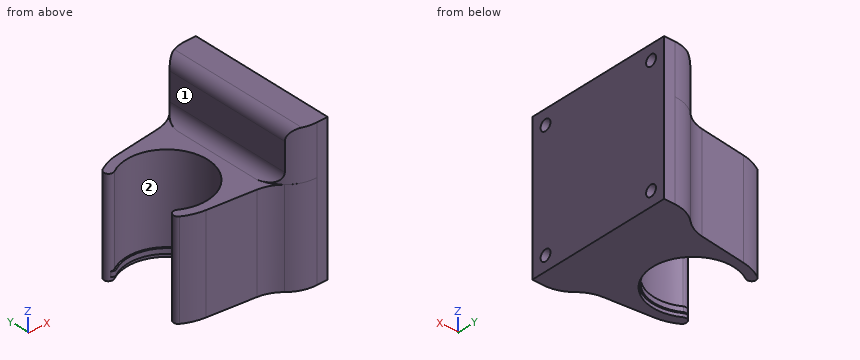
```python
from build123d import *

# Parameters (mm, degrees)
PAD001_DEPTH = 1.4
PAD_DEPTH    = 26.4
PAD002_DEPTH = 13.6
FILLET_R     = 3
SKETCH029_R  = 1.5
POCKET_DEPTH = 7


with BuildPart() as pad001:
    # Sketch001 → Pad001 (new body)
    with BuildSketch(Plane.XY.offset(1)):
        with BuildLine():
            ThreePointArc((-5.627749, -9.1592), (10.75, 0), (-5.627749, 9.1592))
            ThreePointArc((-6.674772, 10.863237), (-7.003279, 9.487707), (-5.627749, 9.1592))
            ThreePointArc((-6.674778, -10.863233), (12.75, -4e-06), (-6.674772, 10.863237))
            ThreePointArc((-5.627749, -9.1592), (-7.003277, -9.487704), (-6.674778, -10.863233))
        make_face()
    extrude(amount=PAD001_DEPTH)


with BuildPart() as mainblock003:
    # Sketch → Pad (new body)
    with BuildSketch(Plane.XY):
        with BuildLine():
            ThreePointArc((-5.837167, -9.499999), (11.15, -4e-06), (-5.83716, 9.500003))
            ThreePointArc((-7.146244, 11.630572), (-7.556981, 9.910749), (-5.83716, 9.500003))
            ThreePointArc((-1.535936, 13.563919), (-4.447417, 12.905792), (-7.146244, 11.630572))
            Line((-1.535936, 13.563919), (11.151047, 15.000553))
            ThreePointArc((11.151047, 15.000553), (14.071423, 15.805596), (16.602936, 17.469367))
            ThreePointArc((23.150107, 20), (19.640497, 19.345319), (16.602936, 17.469367))
            Line((26.150107, 20), (23.150107, 20))
            Line((26.150107, 20), (26.150107, -20))
            Line((26.150107, -20), (23.150107, -20))
            ThreePointArc((16.603443, -17.468808), (19.640708, -19.344966), (23.150107, -20))
            ThreePointArc((16.603443, -17.468808), (14.071743, -15.804671), (11.151047, -14.999447))
            Line((-1.535936, -13.562681), (11.151047, -14.999447))
            ThreePointArc((-7.145609, -11.629518), (-4.447087, -12.904605), (-1.535936, -13.562681))
            ThreePointArc((-5.837167, -9.499999), (-7.556142, -9.910541), (-7.145609, -11.629518))
        make_face()
    extrude(amount=PAD_DEPTH)

    # Sketch005 → Pad002 (new body)
    with BuildSketch(Plane.XY.offset(26.4)):
        with BuildLine():
            ThreePointArc((23.150107, 20), (19.654391, 19.341825), (16.630025, 17.469276))
            Line((16.630025, 17.469276), (16.630025, -17.469302))
            ThreePointArc((16.630025, -17.469302), (19.654393, -19.341837), (23.150107, -20))
            Line((26.150107, -20), (23.150107, -20))
            Line((26.150107, 20), (26.150107, -20))
            Line((26.150107, 20), (23.150107, 20))
        make_face()
    extrude(amount=PAD002_DEPTH)

    # Fillet
    fillet_edges = [mainblock003.edges().sort_by_distance(p)[0] for p in [
        (16.630025, -1.3e-05, 40),
        (16.630025, -1.3e-05, 26.4),
    ]]
    fillet(fillet_edges, radius=FILLET_R)

    # Fusion: union Pad001
    add(pad001.part)


with BuildPart() as mainblock003_1:
    # Fusion placement: moved
    add(mainblock003.part.moved(Location((0, 0, 19.75))))

    # Sketch029 → Pocket (cut)
    with BuildSketch(Plane(origin=(26.150107, 0, 19.75), x_dir=(0, 1, 0), z_dir=(1, 0, 0))):
        with Locations((-16, 36)):
            Circle(SKETCH029_R)
        with Locations((16, 36)):
            Circle(SKETCH029_R)
        with Locations((16, 4)):
            Circle(SKETCH029_R)
        with Locations((-16, 4)):
            Circle(SKETCH029_R)
    extrude(amount=-POCKET_DEPTH, mode=Mode.SUBTRACT)


solid = mainblock003_1.part
```
CAD build for the part. Positions are in the model's coordinates, mm. Face numbers are marked on the shaded views. A direction names the side the tool comes from. Round coordinates to 2 decimals unless told otherwise and drop trailing zeros. Write each loop counter-clockwise with the first axis right and the second up, starting at its lowest first coordinate (ties: lowest second). Pieces come first, ordered by that corner, then holes.
Item 1: Band-saw the part on B-B on y = 0. Write the cut outline in (x, z).
Filled in:
outline: (10.75, 20.75) - (11.15, 20.75) - (11.15, 19.75) - (26.15, 19.75) - (26.15, 59.75) - (19.63, 59.75) arc R3 ccw to (16.63, 56.75) - (16.63, 49.15) arc R3 cw to (13.63, 46.15) - (11.15, 46.15) - (11.15, 22.15) - (10.75, 22.15) - close
Item 2: Drop flat-ended pins along their axis: pin 1 Ø2.5 at (y, z) = (3, 51.5) entering from -X; pin 2 Ø1.8 at (y, z) = (16, 23.75) entering from +X; pin 3 Ø3 at (x, y) = (7.5, 12) entering from +Z. Give the stop position or say it passes through.
Filled in:
pin 1: stops at x = 16.63
pin 2: stops at x = 19.15
pin 3: stops at z = 46.15
Item 3: Drill centre lines: L1, parallel to Z at x = 24, y = 16; L2, parallel to Y at x = 20.5, z = 56; L3, parallel to X at y = 3.5, z = 50.5. Where is each one in solid material? Low to high.
Filled in:
L1: z = 19.75 to 22.25, 25.25 to 54.25, 57.25 to 59.75
L2: y = -19.63 to -17.48, -14.52 to 14.52, 17.48 to 19.63
L3: x = 16.63 to 26.15
Item 4: Tool access for the marked faces 1 and 2: list every direction of +Z, -Z, +X, -X, +Y, -Y with a clear straight run to the whole face (end or side of a thin tool).
Filled in:
face 1: +Z, -X, +Y, -Y
face 2: +Z
Item 5: Band-saw the part on C-C on x = -3.5. Write the cut outline in (y, z).
Filled in:
outline: (-13.19, 19.75) - (-10.59, 19.75) - (-10.59, 20.75) - (-10.16, 20.75) - (-10.16, 22.15) - (-10.59, 22.15) - (-10.59, 46.15) - (-13.19, 46.15) - close; (10.16, 20.75) - (10.59, 20.75) - (10.59, 19.75) - (13.19, 19.75) - (13.19, 46.15) - (10.59, 46.15) - (10.59, 22.15) - (10.16, 22.15) - close
Item 6: Band-saw the part on A-A on z = 55.75. Write the cut outline in (x, y), then the cut area to 3 significant figures.
Filled in:
outline: (16.63, -17.47) arc R9.71 ccw to (23.15, -20) - (26.15, -20) - (26.15, -17.5) - (19.15, -17.5) - (19.15, -14.5) - (26.15, -14.5) - (26.15, 14.5) - (19.15, 14.5) - (19.15, 17.5) - (26.15, 17.5) - (26.15, 20) - (23.15, 20) arc R9.71 ccw to (16.63, 17.47) - close
area: 328 mm2
Item 7: Band-saw the part on D-D on z = 43. Write the cut outline in (x, y), then the cut area to 3 significant figures.
Filled in:
outline: (-7.15, -11.63) arc R13.65 ccw to (-1.54, -13.56) - (11.15, -15) arc R9.73 cw to (16.6, -17.47) arc R9.73 ccw to (23.15, -20) - (26.15, -20) - (26.15, 20) - (23.15, 20) arc R9.73 ccw to (16.6, 17.47) arc R9.73 cw to (11.15, 15) - (-1.54, 13.56) arc R13.65 ccw to (-7.15, 11.63) arc R1.25 ccw to (-5.84, 9.5) arc R11.15 cw (long way) to (-5.84, -9.5) arc R1.25 ccw to start
area: 709 mm2
